from build123d import *

# Parameters (mm, degrees)
SKETCH1_W           = 14
SKETCH1_H           = 14
SKETCH1_W_2         = 13.96
SKETCH1_H_2         = 13.96
SKETCH1_W_3         = 17.83
SKETCH1_H_3         = 34.365
SKETCH1_W_4         = 16.8
SKETCH1_H_4         = 14.955
BOSS_EXTRUDE2_DEPTH = 4
SKETCH3_W           = 14
SKETCH3_H           = 16
CUT_EXTRUDE1_DEPTH  = 2.5
SKETCH6_W           = 145
SKETCH6_H           = 81.124541
BOSS_EXTRUDE3_DEPTH = 8
SKETCH12_R          = 1.25
CUT_EXTRUDE5_DEPTH  = 6
SKETCH13_W          = 18.93
SKETCH13_H          = 35
CUT_EXTRUDE6_DEPTH  = 7
SKETCH14_W          = 16.8
SKETCH14_H          = 14.955
CUT_EXTRUDE8_DEPTH  = 5.75
SKETCH15_R          = 4
CUT_EXTRUDE9_DEPTH  = 10
SKETCH16_R          = 11
CUT_EXTRUDE10_DEPTH = 2.25
SKETCH20_W          = 145
SKETCH20_H          = 81.124541
SKETCH20_W_2        = 130
SKETCH20_H_2        = 66.1
BOSS_EXTRUDE5_DEPTH = 1
SKETCH21_W          = 145
SKETCH21_H          = 34.866824831
CUT_EXTRUDE11_DEPTH = 18
FILLET1_R           = 3
SKETCH28_W          = 11.3
SKETCH28_H          = 2
CUT_EXTRUDE14_DEPTH = 10
SKETCH31_W          = 11.3
SKETCH31_H          = 6
CUT_EXTRUDE15_DEPTH = 16


with BuildPart() as part:
    # Sketch1 → Boss-Extrude2 (new body)
    with BuildSketch(Plane(origin=(0, 0, 0), x_dir=(1, 0, 0), z_dir=(0, 1, 0))):
        Polygon((0, 0), (109.34, 0), (130, 0), (130, 66.1), (0, 66.1), align=None)
        with Locations((51.87, 10.55)):
            Rectangle(SKETCH1_W, SKETCH1_H, mode=Mode.SUBTRACT)
        with Locations((32.81, 10.55)):
            Rectangle(SKETCH1_W, SKETCH1_H, mode=Mode.SUBTRACT)
        with Locations((32.81, 29.6)):
            Rectangle(SKETCH1_W, SKETCH1_H, mode=Mode.SUBTRACT)
        with Locations((32.79, 48.63)):
            Rectangle(SKETCH1_W_2, SKETCH1_H_2, mode=Mode.SUBTRACT)
        with Locations((13.145, 42.2325)):
            Rectangle(SKETCH1_W_3, SKETCH1_H_3, mode=Mode.SUBTRACT)
        with Locations((13.75, 10.55)):
            Rectangle(SKETCH1_W, SKETCH1_H, mode=Mode.SUBTRACT)
        with Locations((51.87, 29.6)):
            Rectangle(SKETCH1_W, SKETCH1_H, mode=Mode.SUBTRACT)
        with Locations((70.93, 10.55)):
            Rectangle(SKETCH1_W, SKETCH1_H, mode=Mode.SUBTRACT)
        with Locations((89.99, 10.55)):
            Rectangle(SKETCH1_W, SKETCH1_H, mode=Mode.SUBTRACT)
        with Locations((117.74, 14.4625)):
            Rectangle(SKETCH1_W_4, SKETCH1_H_4, mode=Mode.SUBTRACT)
        with Locations((70.93, 29.6)):
            Rectangle(SKETCH1_W, SKETCH1_H, mode=Mode.SUBTRACT)
        with Locations((89.99, 29.6)):
            Rectangle(SKETCH1_W, SKETCH1_H, mode=Mode.SUBTRACT)
        with Locations((51.87, 48.65)):
            Rectangle(SKETCH1_W, SKETCH1_H, mode=Mode.SUBTRACT)
        with Locations((70.93, 48.65)):
            Rectangle(SKETCH1_W, SKETCH1_H, mode=Mode.SUBTRACT)
        with Locations((89.99, 48.65)):
            Rectangle(SKETCH1_W, SKETCH1_H, mode=Mode.SUBTRACT)
        with Locations((117.74, 44.7175)):
            Rectangle(SKETCH1_W_4, SKETCH1_H_4, mode=Mode.SUBTRACT)
    extrude(amount=BOSS_EXTRUDE2_DEPTH)

    # Sketch3 → Cut-Extrude1 (cut)
    with BuildSketch(Plane(origin=(0, 0, 0), x_dir=(1, 0, 0), z_dir=(0, 1, 0))):
        with Locations((89.99, 29.6)):
            Rectangle(SKETCH3_W, SKETCH3_H)
        with Locations((70.93, 29.6)):
            Rectangle(SKETCH3_W, SKETCH3_H)
        with Locations((89.99, 48.65)):
            Rectangle(SKETCH3_W, SKETCH3_H)
        with Locations((70.93, 48.65)):
            Rectangle(SKETCH3_W, SKETCH3_H)
        with Locations((51.87, 48.65)):
            Rectangle(SKETCH3_W, SKETCH3_H)
        with Locations((32.81, 48.65)):
            Rectangle(SKETCH3_W, SKETCH3_H)
        with Locations((32.81, 29.650197757)):
            Rectangle(SKETCH3_W, SKETCH3_H)
        with Locations((51.87, 29.6)):
            Rectangle(SKETCH3_W, SKETCH3_H)
        with Locations((13.75, 10.55)):
            Rectangle(SKETCH3_W, SKETCH3_H)
        with Locations((32.81, 10.55)):
            Rectangle(SKETCH3_W, SKETCH3_H)
        with Locations((51.87, 10.55)):
            Rectangle(SKETCH3_W, SKETCH3_H)
        with Locations((70.93, 10.55)):
            Rectangle(SKETCH3_W, SKETCH3_H)
        with Locations((89.99, 10.55)):
            Rectangle(SKETCH3_W, SKETCH3_H)
    extrude(amount=CUT_EXTRUDE1_DEPTH, mode=Mode.SUBTRACT)

    # Sketch6 → Boss-Extrude3 (add)
    with BuildSketch(Plane(origin=(0, 0, 0), x_dir=(-1, 0, 0), z_dir=(0, -1, 0))):
        with Locations((-65, 33.3140765)):
            Rectangle(SKETCH6_W, SKETCH6_H)
        Polygon((-99.99, 58.61), (-39.77, 58.61), (-22.81, 58.61), (-22.81, 53.222321133), (-22.81, 20.55), (-3.75, 20.55), (-3.75, 12.496372948), (-3.75, 0.461789698), (-20.75, 0.461789698), (-99.99, 0.461789698), align=None, mode=Mode.SUBTRACT)
    extrude(amount=-BOSS_EXTRUDE3_DEPTH)

    # Sketch12 → Cut-Extrude5 (cut)
    with BuildSketch(Plane(origin=(0, 0, 0), x_dir=(-1, 0, 0), z_dir=(0, -1, 0))):
        with BuildLine():
            ThreePointArc((-1, 63.85), (-1.366116524, 64.733883476), (-2.25, 65.1))
            Line((-2.25, 65.1), (-2.25, 63.85))
            Line((-2.25, 63.85), (-1, 63.85))
        make_face()
        with BuildLine():
            Line((-2.25, 63.85), (-2.25, 65.1))
            ThreePointArc((-2.25, 65.1), (-3.133883476, 62.966116524), (-1, 63.85))
            Line((-1, 63.85), (-2.25, 63.85))
        make_face()
        with BuildLine():
            ThreePointArc((-1, 2.25), (-3.133883476, 3.133883476), (-2.25, 1))
            Line((-2.25, 1), (-2.25, 2.25))
            Line((-2.25, 2.25), (-1, 2.25))
        make_face()
        with BuildLine():
            Line((-2.25, 2.25), (-2.25, 1))
            ThreePointArc((-2.25, 1), (-1.366116524, 1.366116524), (-1, 2.25))
            Line((-1, 2.25), (-2.25, 2.25))
        make_face()
        with BuildLine():
            ThreePointArc((-129, 2.25), (-128.633883476, 1.366116524), (-127.75, 1))
            Line((-127.75, 1), (-127.75, 2.25))
            Line((-127.75, 2.25), (-129, 2.25))
        make_face()
        with BuildLine():
            Line((-127.75, 2.25), (-127.75, 1))
            ThreePointArc((-127.75, 1), (-126.866116524, 1.366116524), (-126.5, 2.25))
            ThreePointArc((-126.5, 2.25), (-127.75, 3.5), (-129, 2.25))
            Line((-129, 2.25), (-127.75, 2.25))
        make_face()
        with Locations(Location((-127.75, 63.819224339, 0), (0, 0, 90))):
            Circle(SKETCH12_R)
    extrude(amount=-CUT_EXTRUDE5_DEPTH, mode=Mode.SUBTRACT)

    # Sketch13 → Cut-Extrude6 (cut)
    with BuildSketch(Plane.XZ):
        with Locations((13.235, -42.55)):
            Rectangle(SKETCH13_W, SKETCH13_H)
    extrude(amount=-CUT_EXTRUDE6_DEPTH, mode=Mode.SUBTRACT)

    # Sketch14 → Cut-Extrude8 (cut)
    with BuildSketch(Plane.XZ):
        with Locations((117.74, -14.4625)):
            Rectangle(SKETCH14_W, SKETCH14_H)
        with Locations((117.74, -44.7175)):
            Rectangle(SKETCH14_W, SKETCH14_H)
    extrude(amount=-CUT_EXTRUDE8_DEPTH, mode=Mode.SUBTRACT)

    # Sketch15 → Cut-Extrude9 (cut)
    with BuildSketch(Plane.XZ):
        with Locations(Location((117.74, -44.7175, 0), (0, 0, 270))):
            Circle(SKETCH15_R)
        with Locations(Location((117.74, -14.4625, 0), (0, 0, 270))):
            Circle(SKETCH15_R)
    extrude(amount=-CUT_EXTRUDE9_DEPTH, mode=Mode.SUBTRACT)

    # Sketch16 → Cut-Extrude10 (cut)
    with BuildSketch(Plane(origin=(0, 8, 0), x_dir=(1, 0, 0), z_dir=(0, 1, 0))):
        with Locations(Location((117.74, 44.7175, 0), (0, 0, 270))):
            Circle(SKETCH16_R)
        with Locations(Location((117.74, 14.4625, 0), (0, 0, 270))):
            Circle(SKETCH16_R)
    extrude(amount=-CUT_EXTRUDE10_DEPTH, mode=Mode.SUBTRACT)

    # Sketch20 → Boss-Extrude5 (add)
    with BuildSketch(Plane.XZ):
        with Locations((65, -33.3140765)):
            Rectangle(SKETCH20_W, SKETCH20_H)
        with Locations((65, -33.05)):
            Rectangle(SKETCH20_W_2, SKETCH20_H_2, mode=Mode.SUBTRACT)
    extrude(amount=BOSS_EXTRUDE5_DEPTH)

    # Sketch21 → Cut-Extrude11 (cut)
    with BuildSketch(Plane(origin=(0, -1.861896279, 0.228612117), x_dir=(-1, 0, 0), z_dir=(0, 0.9925461516413211, -0.1218693434051548))):
        with Locations((-65, 24.505710134)):
            Rectangle(SKETCH21_W, SKETCH21_H)
    extrude(amount=CUT_EXTRUDE11_DEPTH, mode=Mode.SUBTRACT)

    # Fillet1
    fillet1_edges = [part.edges().sort_by_distance(p)[0] for p in [
        (-7.5, 3.5, 6.695663476),
        (137.5, 3.5, 6.695663476),
    ]]
    fillet(fillet1_edges, radius=FILLET1_R)

    # Sketch28 → Cut-Extrude14 (cut)
    with BuildSketch(Plane.XZ):
        Polygon((16.91, -59.36), (16.91, -55.61), (16.91, -54.36), (9.61, -54.36), (9.61, -59.36), align=None)
        with Locations((13.26, -60.36)):
            Rectangle(SKETCH28_W, SKETCH28_H)
    extrude(amount=-CUT_EXTRUDE14_DEPTH, mode=Mode.SUBTRACT)

    # Sketch31 → Cut-Extrude15 (cut)
    with BuildSketch(Plane.XY.offset(-61.36)):
        with Locations((13.26, 5)):
            Rectangle(SKETCH31_W, SKETCH31_H)
    extrude(amount=-CUT_EXTRUDE15_DEPTH, mode=Mode.SUBTRACT)


solid = part.part
Can you work these out from the model? Positions are in its coordinate system, mm. A direction names the side the tool comes from. Round coordinates to 2 decimals unless told otherwise and drop trailing zeros. Write each loop counter-clockwise with the first axis right and the second up, starting at its lowest first coordinate (ties: lowest second). Pieces come first, ordered by that corner, then holes. Notation, with made-up numbers: M 27,-25.5 L 85,-25.5 A19 cw 85,-7.5 Z; hole C 13.5,-2.5 d8. An arc over 180 degrees is marked long. Use a Markdown table: item, result.
Item 1: I want a section at C-C (x = 62). List the corners of the cut face in (y, z) for me, and give its area (3 significant figures).
Found:
| item | result |
|---|---|
| outline | M -1,-73.88 L 8,-73.88 L 8,-58.61 L 4,-58.61 L 4,-0.46 L 8,-0.46 L 8,6.14 L -1,7.25 L -1,0 L 0,0 L 0,-66.1 L -1,-66.1 Z |
| area | 426 mm2 |
Item 2: For pin 1 Ø1.2 at (x, y) = (50, 3.5) entering from +Z; pin 2 Ø4 at (x, y) = (13.5, 5.5) entering from +Z; pin 3 Ø0.8 at (x, y) = (36, 1) entering from +Z, each with a flat end and sliding along its axis, tell me the tip position at first contact or that it passes through.
Found:
| item | result |
|---|---|
| pin 1 | stops at z = 6.77 |
| pin 2 | stops at z = 6.7 |
| pin 3 | stops at z = 7.05 |
Item 3: We'd pull the mould along X, two halves only. Please class faces 3 (the face through (137.5, 4, -35)), 4 (the face through (58.87, 2, -10)), 5 (the face through (-6.645, 3.638, 5.77)): released by +X, released by -X, zero draft, split by the parting line, or undercut.
Found:
| item | result |
|---|---|
| face 3 | released by +X |
| face 4 | undercut |
| face 5 | released by -X |
Item 4: I want a section at A-A (x = 117.74). State how many separate pieces and enclosed holes the cut face has, and give its area (3 significant figures).
Found:
| item | result |
|---|---|
| separate pieces | 3 |
| enclosed holes | 0 |
| area | 388 mm2 |
Item 5: If I drill on line 1 along X through (y, z) = (3.75, -63.85); line 2 along X through (y, z) = (0.25, -27); line 3 along X through (y, z) = (1.25, -40), over which ranges is the centre line in solid material (lowest first)? Write a range as [from, to].
Found:
| item | result |
|---|---|
| line 1 | x = [-7.5, 1], [3.5, 7.61], [18.91, 126.5], [129, 137.5] |
| line 2 | x = [-7.5, 3.77], [22.7, 25.81], [39.81, 44.87], [58.87, 63.93], [77.93, 82.99], [96.99, 137.5] |
| line 3 | x = [-7.5, 3.77], [22.7, 109.34], [126.14, 137.5] |
Item 6: Which directions (+Z, -Z, +X, -X, +Y, -Y) give clear straight access to the entire face, cutting with the end or side of a thin tool? Please do faces 1 (the face through (25.81, 2, -49)), 2 (the face through (-7.5, 4, -35)).
Found:
| item | result |
|---|---|
| face 1 | -Y |
| face 2 | +Z, -Z, -X, +Y, -Y |
Item 7: I want a section at D-D (x = 11). List the corners of the cut face in (y, z) for me.
Found:
| item | result |
|---|---|
| outline | M -1,-73.88 L 2,-73.88 L 2,-61.36 L 0,-61.36 L 0,-66.1 L -1,-66.1 Z; M -1,0 L 0,0 L 0,-2.55 L 2.5,-2.55 L 2.5,-3.55 L 4,-3.55 L 4,-0.46 L 8,-0.46 L 8,6.14 L -1,7.25 Z; M 0,-25.05 L 7,-25.05 L 7,-54.36 L 8,-54.36 L 8,-20.55 L 4,-20.55 L 4,-17.55 L 2.5,-17.55 L 2.5,-18.55 L 0,-18.55 Z |
